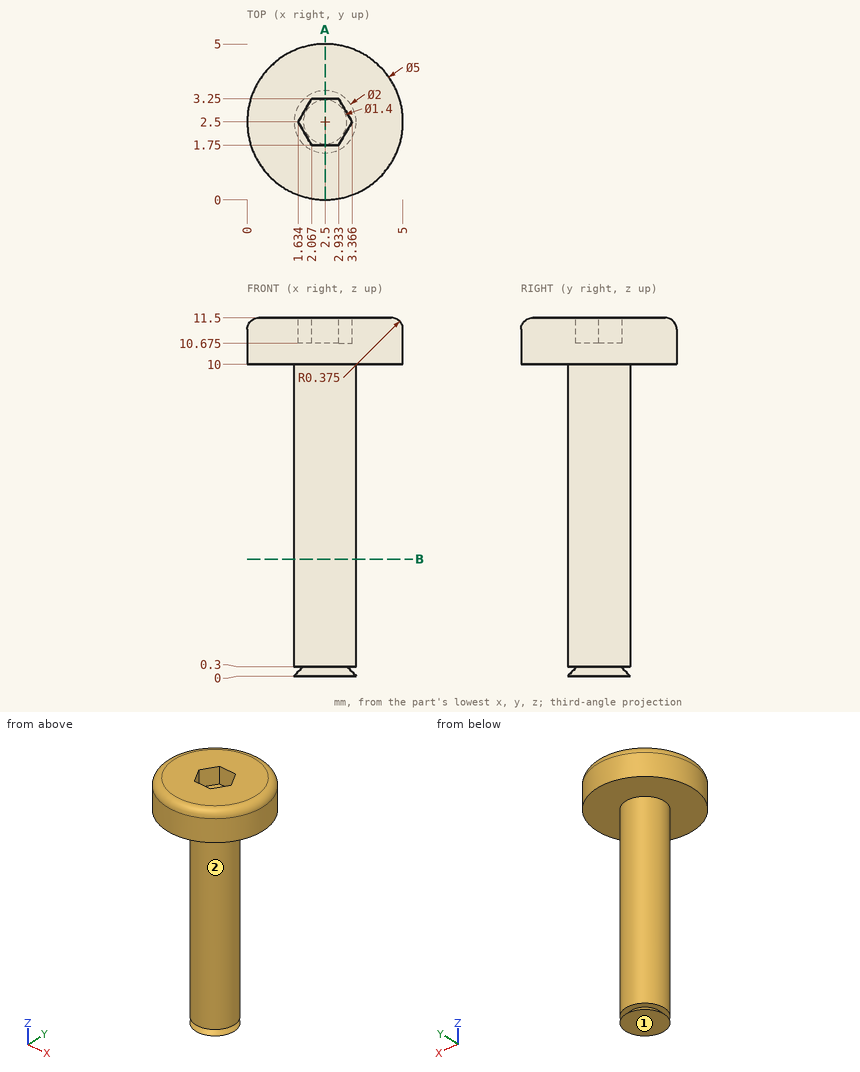
Could you check a few things on this drawing? It's one solid part, dimensions in mm from its lowest x, y, z. A direction names the side the tool comes from. Give positions to 0.01 mm unless a question says otherwise; leave off trailing zeros. Order: outer loops, then holes, each group sorted by start corner. A loop starts at its lowest first (then second) coordinate and runs counter-clockwise, first axis right, second up. Notation, with made-up numbers: (8.25, 56.25) - (23.25, 56.25) arc R5 cw to (23.25, 64.25) - close; hole circle Ø6 at (45.25, -33.75). An arc over 180 degrees is marked (long way). Return JSON: item names as keys, results as strings. Group by question number.
Q1. Suppose I cut it at B-B, the plane z = 3.75. Please give me the cut outline in (x, y).
Q2. Please list where these lines run through material, in increasing order: line 1 along Z through (x, y) = (1.55, 3.35); line 2 along Y through (x, z) = (2.45, 3.5). Write a range as [from, to].
Q3. Suppose I cut it at A-A, the plane x = 2.5. Please give me the cut outline in (y, z) (3 decimals), and give its area (3 significant figures).
Q4. Which directions (+Z, -Z, +X, -X, +Y, -Y) give clear straight access to the entire face, cutting with the end or side of a thin tool? Please do the marked faces 1 and 2.
Q5. Will this pin go through, and if not, where does the flat tip stop? pin 1 Ø1.5 at (y, z) = (2, 2.5) entering from -X.
Resolved:
{
 "1": {"outline": "circle Ø2 at (2.5, 2.5)"},
 "2": {"line 1": "z = [10, 11.5]", "line 2": "y = [1.5, 3.5]"},
 "3": {"outline": "(0, 10) - (1.5, 10) - (1.5, 0.3) - (1.8, 0.3) - (1.5, 0) - (3.5, 0) - (3.2, 0.3) - (3.5, 0.3) - (3.5, 10) - (5, 10) - (5, 11.125) arc R0.375 ccw to (4.625, 11.5) - (3.25, 11.5) - (3.25, 10.675) - (1.75, 10.675) - (1.75, 11.5) - (0.375, 11.5) arc R0.375 ccw to (0, 11.125) - close", "area": "26.1 mm2"},
 "4": {"face 1": "-Z, +X, -X, +Y, -Y", "face 2": "-Z"},
 "5": {"pin 1": "stops at x = 1.5"}
}
